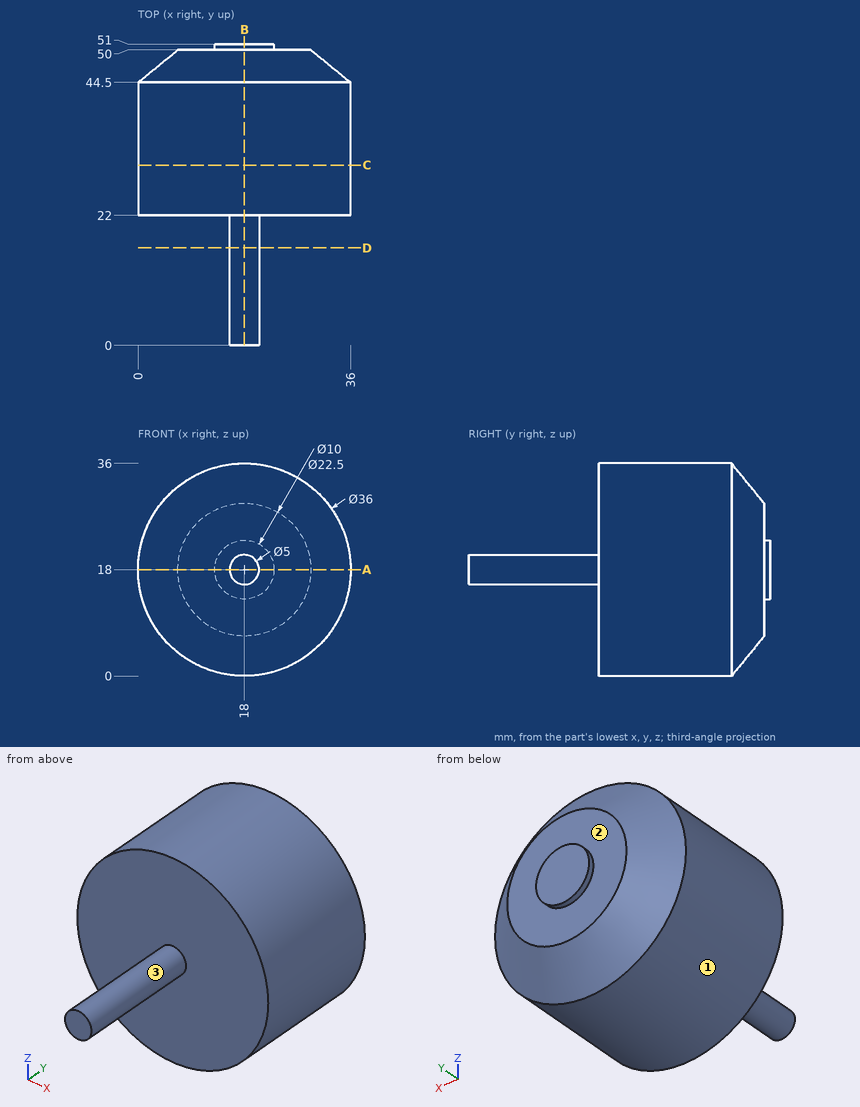
Print and shaded views of the part. All mm, measured from the part's lowest x, y and z. A direction names the side the tool comes from. Give positions to 0.01 mm unless a question says otherwise; leave off trailing zeros. Write each loop counter-clockwise with the first axis right and the second up, starting at its lowest first coordinate (ties: lowest second). Pieces come first, ordered by that corner, then holes. Notation, with made-up numbers: (26.25, -5.5) - (38.25, -5.5) arc R23 ccw to (38.25, 30.5) - close; hole circle Ø7 at (63, 52.5). An arc over 180 degrees is marked (long way). One line per question, with ' | ' between items. Start each with the question number.
(1) Slice it at A-A on z = 18. Write the cut outline in (x, y), plus the area to 3 significant figures.
(2) Slice it at C-C on y = 30.5. Write the cut outline in (x, z), plus the area to 3 significant figures.
(3) Slice it at B-B on x = 18. Write the cut outline in (y, z), plus the area to 3 significant figures.
(4) Slice it at D-D on y = 16.5. Write the cut outline in (x, z).
(5) Wall check: line 1 along Y through (x, z) = (16.5, 24); line 2 along Y through (x, z) = (15.5, 17); line 3 along Z through (x, y) = (6.5, 36). Give the ranges that are in metal, low to high. Write a range as from..to.
(6) 3-axis set-ups, long thin cutter, end or side, ignore diameter. For the marked faces 1, 2 and 3: which of +Z, -Z, +X, -X, +Y, -Y reach the whole face in a straight line?
(7) Pin check, flat tips, straight feed: P1, Ø8, axis at x = 13.5, y = 45.5, coming from the -Z side; P2, Ø1.5, axis at x = 17, z = 22, coming from the -Y side; P3, Ø3, axis at y = 43.5, z = 29.5, coming from the -X side. Stop position of each tip, or through.
Results below:
1) outline: (0, 22) - (15.5, 22) - (15.5, 0) - (20.5, 0) - (20.5, 22) - (36, 22) - (36, 44.5) - (29.25, 50) - (23, 50) - (23, 51) - (13, 51) - (13, 50) - (6.75, 50) - (0, 44.5) - close | area: 1,090 mm^2
2) outline: circle Ø36 at (18, 18) | area: 1,020 mm^2
3) outline: (0, 15.5) - (22, 15.5) - (22, 0) - (44.5, 0) - (50, 6.75) - (50, 13) - (51, 13) - (51, 23) - (50, 23) - (50, 29.25) - (44.5, 36) - (22, 36) - (22, 20.5) - (0, 20.5) - close | area: 1,090 mm^2
4) outline: circle Ø5 at (18, 18)
5) line 1: 22..50 | line 2: 22..51 | line 3: 4.15..31.85
6) face 1: +Y, -Y | face 2: +Y | face 3: -Y
7) P1: z = 0.01 | P2: y = 22 | P3: x = 3.03
